The listing builds one solid part. Answer for the finished solid, in the listing's coordinates (mm). A direction names the side the tool comes from. Round coordinates to 2 decimals unless told otherwise and drop trailing zeros. Write each loop counter-clockwise with the first axis right and the second up, starting at its lowest first coordinate (ties: lowest second). Pieces come first, ordered by that corner, then holes.
from build123d import *

# Parameters (mm, degrees)
SKETCH1_R                = 1.5
BOSS_EXTRUDE1_DEPTH      = 9.22
BOSS_EXTRUDE2_DEPTH      = 12
SHELL1_START             = -10
SHELL1_OUTLINE_W         = 20.5
SHELL1_OUTLINE_H         = 16.44
SHELL1_DEPTH             = 27.5
SHELL1_START_2           = -29.5
SHELL1_2_DEPTH           = 14.5
SHELL1_START_3           = -16.5
SHELL1_3_DEPTH           = 1.5
SHELL1_START_4           = -8.22
SHELL1_4_DEPTH           = 16.44
SKETCH3_R                = 1.5
BOSS_EXTRUDE3_DEPTH      = 1
BOSS_EXTRUDE4_DEPTH      = 1.5
BOSS_EXTRUDE4_DEPTH_BACK = 1.5
SKETCH6_W                = 5
SKETCH6_H                = 5
SKETCH6_R                = 1.5
SKETCH7_R                = 2.75
CUT_EXTRUDE1_DEPTH       = 37.562906066
FILLET1_R                = 1
CUT_EXTRUDE2_DEPTH       = 20
CUT_EXTRUDE2_DEPTH_BACK  = 20
SKETCH8_R                = 0.956029162


with BuildPart() as part:
    # Sketch1 → Boss-Extrude1 (new, symmetric)
    with BuildSketch(Plane.XY):
        with BuildLine():
            Line((17.5, -11.25), (-17.5, -11.25))
            Line((-17.5, -11.25), (-17.5, 11.25))
            Line((-17.5, 11.25), (17.5, 11.25))
            ThreePointArc((17.5, 11.25), (18.914213562, 10.664213562), (19.5, 9.25))
            Line((19.5, 9.25), (19.5, -9.25))
            ThreePointArc((19.5, -9.25), (18.914213562, -10.664213562), (17.5, -11.25))
        make_face()
        with Locations((-12.5, 8.75)):
            Circle(SKETCH1_R, mode=Mode.SUBTRACT)
        with Locations((-12.5, -8.75)):
            Circle(SKETCH1_R, mode=Mode.SUBTRACT)
    extrude(amount=BOSS_EXTRUDE1_DEPTH, both=True)

    # Sketch2 → Boss-Extrude2 (add)
    with BuildSketch(Plane.ZY.offset(17.5)):
        with BuildLine():
            Line((9.22, -7.5), (9.22, 7.5))
            ThreePointArc((9.22, 7.5), (0, 11.25), (-9.22, 7.5))
            Line((-9.22, 7.5), (-9.22, -7.5))
            ThreePointArc((-9.22, -7.5), (0, -11.25), (9.22, -7.5))
        make_face()
    extrude(amount=BOSS_EXTRUDE2_DEPTH)

    # Shell1: read off the stored shape, not the designer's step
    # Shell1 outline → Shell1 (cut)
    with BuildSketch(Plane.YZ.offset(SHELL1_START)):
        Rectangle(SHELL1_OUTLINE_W, SHELL1_OUTLINE_H)
    extrude(amount=SHELL1_DEPTH, mode=Mode.SUBTRACT)

    # Shell1 2 outline → Shell1 2 (cut)
    with BuildSketch(Plane.YZ.offset(SHELL1_START_2)):
        with BuildLine():
            ThreePointArc((7.068411902, -8.22), (10.25, 0), (7.068411902, 8.22))
            Line((7.068411902, 8.22), (-7.068411902, 8.22))
            ThreePointArc((-7.068411902, 8.22), (-10.25, 0), (-7.068411902, -8.22))
            Line((-7.068411902, -8.22), (7.068411902, -8.22))
        make_face()
    extrude(amount=SHELL1_2_DEPTH, mode=Mode.SUBTRACT)

    # Shell1 3 outline → Shell1 3 (cut)
    with BuildSketch(Plane.YZ.offset(SHELL1_START_3)):
        with BuildLine():
            Line((10.25, 0), (10.25, 8.22))
            Line((10.25, 8.22), (7.068411902, 8.22))
            ThreePointArc((7.068411902, 8.22), (9.426855331, 4.407122157), (10.25, 0))
        make_face()
        with BuildLine():
            Line((10.25, -8.22), (10.25, 0))
            ThreePointArc((10.25, 0), (9.426855331, -4.407122157), (7.068411902, -8.22))
            Line((7.068411902, -8.22), (10.25, -8.22))
        make_face()
        with BuildLine():
            ThreePointArc((-10.25, 0), (-9.426855331, 4.407122157), (-7.068411902, 8.22))
            Line((-7.068411902, 8.22), (-10.25, 8.22))
            Line((-10.25, 8.22), (-10.25, 0))
        make_face()
        with BuildLine():
            Line((-10.25, -8.22), (-7.068411902, -8.22))
            ThreePointArc((-7.068411902, -8.22), (-9.426855331, -4.407122157), (-10.25, 0))
            Line((-10.25, 0), (-10.25, -8.22))
        make_face()
    extrude(amount=SHELL1_3_DEPTH, mode=Mode.SUBTRACT)

    # Shell1 4 outline → Shell1 4 (cut)
    with BuildSketch(Plane.XY.offset(SHELL1_START_4)):
        with BuildLine():
            ThreePointArc((-14.5, -10.25), (-14.871708245, -9.540569415), (-15, -8.75))
            Line((-15, -8.75), (-15, -10.25))
            Line((-15, -10.25), (-14.5, -10.25))
        make_face()
        with BuildLine():
            ThreePointArc((-10, 8.75), (-12.499999993, 6.25), (-15, 8.749999987))
            Line((-15, 8.749999987), (-15, -8.75))
            ThreePointArc((-15, -8.75), (-12.5, -6.25), (-10, -8.75))
            Line((-10, -8.75), (-10, 8.75))
        make_face()
        with BuildLine():
            Line((-14.5, 10.25), (-15, 10.25))
            Line((-15, 10.25), (-15, 8.749999987))
            ThreePointArc((-15, 8.749999987), (-14.871708247, 9.540569409), (-14.5, 10.25))
        make_face()
        with BuildLine():
            ThreePointArc((-10.5, 10.25), (-10.128291755, 9.540569415), (-10, 8.75))
            Line((-10, 8.75), (-10, 10.25))
            Line((-10, 10.25), (-10.5, 10.25))
        make_face()
        with BuildLine():
            Line((-10, -10.25), (-10, -8.75))
            ThreePointArc((-10, -8.75), (-10.128291755, -9.540569415), (-10.5, -10.25))
            Line((-10.5, -10.25), (-10, -10.25))
        make_face()
        with BuildLine():
            ThreePointArc((18.5, 9.25), (18.207106781, 9.957106781), (17.5, 10.25))
            Line((17.5, 10.25), (17.5, -10.25))
            ThreePointArc((17.5, -10.25), (18.207106781, -9.957106781), (18.5, -9.25))
            Line((18.5, -9.25), (18.5, 9.25))
        make_face()
    extrude(amount=SHELL1_4_DEPTH, mode=Mode.SUBTRACT)

    # Sketch3 → Boss-Extrude3 (add)
    with BuildSketch(Plane.ZY.offset(17.5)):
        with BuildLine():
            Line((-9.22, 7.5), (-9.22, -7.5))
            ThreePointArc((-9.22, -7.5), (0, -11.25), (9.22, -7.5))
            Line((9.22, -7.5), (9.22, 7.5))
            ThreePointArc((9.22, 7.5), (0, 11.25), (-9.22, 7.5))
        make_face()
        Circle(SKETCH3_R, mode=Mode.SUBTRACT)
    extrude(amount=BOSS_EXTRUDE3_DEPTH)

    # Sketch6 → Boss-Extrude4 (add, two sides: drawn at the far end of the back side and taken through both)
    with BuildSketch(Plane.XY.offset(-0.58).offset(-BOSS_EXTRUDE4_DEPTH_BACK)):
        with Locations((22, 0)):
            Rectangle(SKETCH6_W, SKETCH6_H)
        with Locations((22, 0)):
            Circle(SKETCH6_R, mode=Mode.SUBTRACT)
    extrude(amount=BOSS_EXTRUDE4_DEPTH + BOSS_EXTRUDE4_DEPTH_BACK)

    # Sketch7 → Cut-Extrude1 (cut, through all)
    with BuildSketch(Plane.XY.offset(9.22)):
        with Locations((7.5, 0)):
            Circle(SKETCH7_R)
    extrude(amount=-CUT_EXTRUDE1_DEPTH, mode=Mode.SUBTRACT)

    # Fillet1
    fillet1_edges = [part.edges().sort_by_distance(p)[0] for p in [
        (19.5, 2.5, -0.58),
        (19.5, -2.5, -0.58),
    ]]
    fillet(fillet1_edges, radius=FILLET1_R)

    # Sketch8 → Cut-Extrude2 (cut, two sides: drawn at the far end of the back side and taken through both)
    with BuildSketch(Plane.XY.offset(-0.58).offset(-CUT_EXTRUDE2_DEPTH_BACK)):
        with Locations(Location((-16.061963922, 9.293970838, 0), (0, 0, 242.73008166))):
            Circle(SKETCH8_R)
        with Locations(Location((-16.061963922, -9.293970838, 0), (0, 0, 242.730056197))):
            Circle(SKETCH8_R)
    extrude(amount=CUT_EXTRUDE2_DEPTH + CUT_EXTRUDE2_DEPTH_BACK, mode=Mode.SUBTRACT)


solid = part.part
1. For a pull along X with two mould halves and no side action, classify faces 1 (the face through (-5, 0, -9.22)), 2 (the face through (18.215, 9.949, -0.115)), 3 (the face through (24.5, 0, -1)) as released by +X, released by -X, zero draft, split by the parting line, or undercut.
Geometry says:
face 1: zero draft
face 2: undercut
face 3: released by +X
2. A tool of negligible diameter and unlimited length cuts with its end or side. For faces 4 (the face through (-17.5, 10, 7)), 5 (the face through (18.5, 0, 0)), 6 (the face through (-24, 0, -8.22)), from which of +Z, -Z, +X, -X, +Y, -Y can it reach the whole face along a straight path? Write none if from no direction.
Geometry says:
face 4: +Z, -X, +Y
face 5: none
face 6: -X
3. Section C-C on y = 0 is taken. Give the number of separate pieces and of enclosed holes in the cut face, plus the area to 3 significant figures.
Geometry says:
separate pieces: 4
enclosed holes: 0
area: 123 mm2
4. Section A-A on x = 22 is taken. Determine the outline of the cut face in (y, z).
Geometry says:
outline: (-2.5, -2.08) - (-1.5, -2.08) - (-1.5, 0.92) - (-2.5, 0.92) - close; (1.5, -2.08) - (2.5, -2.08) - (2.5, 0.92) - (1.5, 0.92) - close
5. Section D-D on x = 4 is taken. Determine the outline of the cut face in (y, z), plus the area to 3 significant figures.
Geometry says:
outline: (-11.25, -9.22) - (11.25, -9.22) - (11.25, 9.22) - (-11.25, 9.22) - close; hole (-10.25, -8.22) - (10.25, -8.22) - (10.25, 8.22) - (-10.25, 8.22) - close
area: 77.9 mm2
6. Straight lines are drawn through the part: line 1 along X through (y, z) = (-5, -4.5); line 2 along Z through (x, y) = (-3.5, -4.75); line 3 along X through (y, z) = (7.5, 6). For each, find the intervals that lie inside material, in ascending order.
Geometry says:
line 1: x = -18.5 to -17.5, 18.5 to 19.5
line 2: z = -9.22 to -8.22, 8.22 to 9.22
line 3: x = -18.5 to -17.5, -14.67 to -13.33, -11.67 to -10.33, 18.5 to 19.5
7. Given pin 1 (1.5 mm diameter, centred on y = 2.5, z = -5.5, fed in from -X); pin 2 (2.5 mm diameter, centred on x = 21.5, y = 1.5, fed in from +Z); pin 3 (3.5 mm diameter, centred on x = 22, y = 0, fed in from -Z), each flat-ended and moving along its own axis, determine where each tip first touches the part or whether it passes through.
Geometry says:
pin 1: stops at x = -18.5
pin 2: stops at z = 0.92
pin 3: stops at z = -2.08
8. Section B-B on y = 4.5 is taken. Determine the outline of the cut face in (x, z), plus the area to 3 significant figures.
Geometry says:
outline: (-29.5, -9.22) - (19.5, -9.22) - (19.5, 9.22) - (-29.5, 9.22) - (-29.5, 8.22) - (-18.5, 8.22) - (-18.5, -8.22) - (-29.5, -8.22) - close; hole (-17.5, -8.22) - (18.5, -8.22) - (18.5, 8.22) - (-17.5, 8.22) - close
area: 131 mm2
